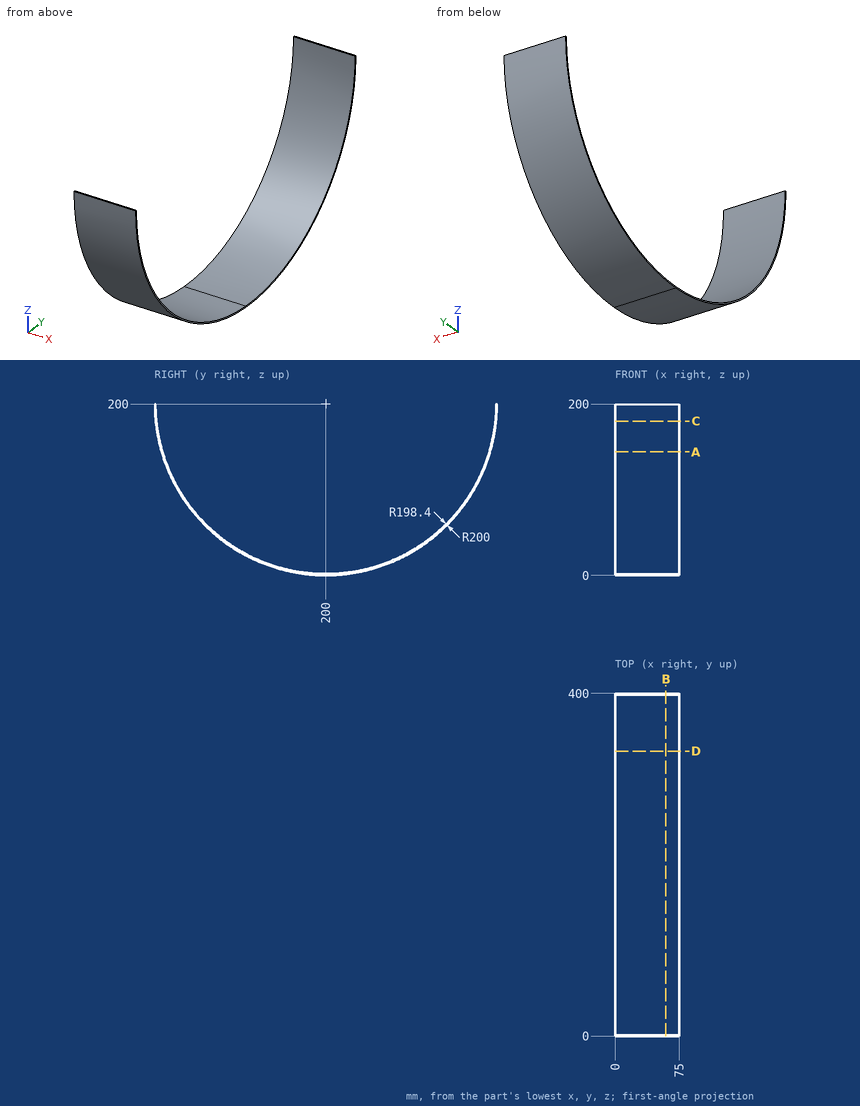
Geometry check sheet. Reference: drawing and pictorial views, mm from the part's lowest x, y, z. Round coordinates to 2 decimals unless told otherwise and drop trailing zeros. Loops run counter-clockwise (first coordinate to the right, second up) from the corner with the lowest first, then second, coordinate; pieces in that order, holes last.
1. Sectioned sample at B-B on x = 59. Record the boundary of the cut face in (y, z), and give its area (3 significant figures).
2. Sectioned sample at C-C on z = 180. Record the boundary of the cut face in (x, y), and give its area (3 significant figures).
3. Scan lines: probe 1 along Y at (x, z) = (55.5, 104); probe 2 along Y at (x, z) = (53, 132); probe 3 along Z at (x, y) = (3.5, 155.5). Record each from-to range of solid material in increasing order.
4. Sectioned sample at D-D on y = 332.5. Record the boundary of the cut face in (x, z), and give its area (3 significant figures).
5. Sectioned sample at A-A on z = 144. Record the boundary of the cut face in (x, y).
6. Gauge pin test, flat ends, axial feed: pin 1 Ø4 at (x, z) = (28.5, 61) entering from +Y; pin 2 Ø6 at (x, z) = (67.5, 26.5) entering from -Y; pin 3 Ø4 at (x, z) = (16.5, 40.5) entering from +Y. Record the tip position at first contact, or that the pin passes through.
Recorded:
1. outline: (0, 200) arc R200 ccw to (400, 200) - (398.4, 200) arc R198.4 cw to (1.6, 200) - close
1. area: 1,000 mm2
2. outline: (0, 1) - (75, 1) - (75, 2.61) - (0, 2.61) - close; (0, 397.39) - (75, 397.39) - (75, 399) - (0, 399) - close
2. area: 241 mm2
3. probe 1: y = 24.55 to 26.37, 373.63 to 375.45
3. probe 2: y = 11.91 to 13.62, 386.38 to 388.09
3. probe 3: z = 5.01 to 6.65
4. outline: (0, 50.19) - (75, 50.19) - (75, 52.33) - (0, 52.33) - close
4. area: 161 mm2
5. outline: (0, 8) - (75, 8) - (75, 9.67) - (0, 9.67) - close; (0, 390.33) - (75, 390.33) - (75, 392) - (0, 392) - close
6. pin 1: stops at y = 345.71
6. pin 2: stops at y = 95.45
6. pin 3: stops at y = 323.26
